Geometry: final body of the model. Coordinates: model frame, mm. A direction names the side the tool comes from. Coordinates: 2 decimals unless noted, no trailing zeros. Order: outer loops, then holes, each group sorted by start corner. A loop starts at its lowest first (then second) coordinate and runs counter-clockwise, first axis right, second up. Notation, with made-up numbers: (-2.5, 44) - (5.5, 44) arc R13 cw to (5.5, 53) - close; hole circle Ø2 at (-2, 47). An arc over 180 degrees is marked (long way). Use a Markdown table: item, result. Add a question column.
```python
from build123d import *

# Parameters (mm, degrees)
SKETCH1_W           = 182
SKETCH1_H           = 137.36
BOSS_EXTRUDE1_DEPTH = 3
SKETCH2_R           = 1.5
CUT_EXTRUDE1_DEPTH  = 4
SKETCH3_R           = 1
CUT_EXTRUDE2_DEPTH  = 4
SKETCH4_W           = 23
SKETCH4_H           = 12.5
CUT_EXTRUDE3_DEPTH  = 4
SKETCH5_R           = 1.35
CUT_EXTRUDE4_DEPTH  = 4
SKETCH6_R           = 1.5
CUT_EXTRUDE5_DEPTH  = 4
CUT_EXTRUDE6_DEPTH  = 4
FILLET1_R           = 7
SKETCH10_R          = 1.5
CUT_EXTRUDE9_DEPTH  = 4
SKETCH11_R          = 1.5
CUT_EXTRUDE10_DEPTH = 4
CUT_EXTRUDE11_REACH = 5
SKETCH13_W          = 12.5
SKETCH13_H          = 23
SKETCH14_R          = 1
CUT_EXTRUDE12_DEPTH = 4
SKETCH15_R          = 2
CUT_EXTRUDE13_DEPTH = 4
SKETCH16_R          = 1.5
CUT_EXTRUDE14_DEPTH = 4


with BuildPart() as part:
    # Sketch1 → Boss-Extrude1 (new body)
    with BuildSketch(Plane(origin=(0, 0, 0), x_dir=(1, 0, 0), z_dir=(0, 1, 0))):
        with Locations((8.068181818, 1013.883570356)):
            Rectangle(SKETCH1_W, SKETCH1_H)
    extrude(amount=BOSS_EXTRUDE1_DEPTH)

    # Sketch2 → Cut-Extrude1 (cut, through all)
    with BuildSketch(Plane.XZ):
        with Locations((95.068181818, -1029.883570356)):
            Circle(SKETCH2_R)
        with Locations((95.068181818, -997.883570356)):
            Circle(SKETCH2_R)
    extrude(amount=-CUT_EXTRUDE1_DEPTH, mode=Mode.SUBTRACT)

    # Sketch3 → Cut-Extrude2 (cut, through all)
    with BuildSketch(Plane(origin=(0, 3, 0), x_dir=(1, 0, 0), z_dir=(0, 1, 0))):
        with Locations((27.328181818, 1076.423570356)):
            Circle(SKETCH3_R)
        with Locations((-0.871818182, 1076.423570356)):
            Circle(SKETCH3_R)
        with Locations((-0.871818182, 951.363570356)):
            Circle(SKETCH3_R)
        with Locations((27.328181818, 951.363570356)):
            Circle(SKETCH3_R)
    extrude(amount=-CUT_EXTRUDE2_DEPTH, mode=Mode.SUBTRACT)

    # Sketch4 → Cut-Extrude3 (cut, through all)
    with BuildSketch(Plane(origin=(0, 3, 0), x_dir=(1, 0, 0), z_dir=(0, 1, 0))):
        with Locations((13.268181818, 951.453570356)):
            Rectangle(SKETCH4_W, SKETCH4_H)
        with Locations((13.268181818, 1076.313570356)):
            Rectangle(SKETCH4_W, SKETCH4_H)
    extrude(amount=-CUT_EXTRUDE3_DEPTH, mode=Mode.SUBTRACT)

    # Sketch5 → Cut-Extrude4 (cut, through all)
    with BuildSketch(Plane.XZ):
        with Locations((77.568181818, -1038.383570356)):
            Circle(SKETCH5_R)
        with Locations((77.668181818, -989.343570356)):
            Circle(SKETCH5_R)
        with Locations((19.568181818, -1038.383570356)):
            Circle(SKETCH5_R)
        with Locations((19.568181818, -989.383570356)):
            Circle(SKETCH5_R)
    extrude(amount=-CUT_EXTRUDE4_DEPTH, mode=Mode.SUBTRACT)

    # Sketch6 → Cut-Extrude5 (cut, through all)
    with BuildSketch(Plane(origin=(0, 3, 0), x_dir=(1, 0, 0), z_dir=(0, 1, 0))):
        with Locations((18.062803793, 1049.383570356)):
            Circle(SKETCH6_R)
        with Locations((-31.937196207, 1049.383570356)):
            Circle(SKETCH6_R)
        with Locations((-31.937196207, 978.387370356)):
            Circle(SKETCH6_R)
        with Locations((18.062803793, 978.387370356)):
            Circle(SKETCH6_R)
    extrude(amount=-CUT_EXTRUDE5_DEPTH, mode=Mode.SUBTRACT)

    # Sketch7 → Cut-Extrude6 (cut, through all)
    with BuildSketch(Plane(origin=(0, 3, 0), x_dir=(1, 0, 0), z_dir=(0, 1, 0))):
        with BuildLine():
            Line((49.068181818, 1063.883570356), (60.068181818, 1063.883570356))
            ThreePointArc((60.068181818, 1063.883570356), (61.482395381, 1063.297783918), (62.068181818, 1061.883570356))
            Line((62.068181818, 1061.883570356), (62.068181818, 965.883570356))
            ThreePointArc((62.068181818, 965.883570356), (61.482395381, 964.469356794), (60.068181818, 963.883570356))
            Line((60.068181818, 963.883570356), (49.068181818, 963.883570356))
            ThreePointArc((49.068181818, 963.883570356), (47.653968256, 964.469356794), (47.068181818, 965.883570356))
            Line((47.068181818, 965.883570356), (47.068181818, 1061.883570356))
            ThreePointArc((47.068181818, 1061.883570356), (47.653968256, 1063.297783918), (49.068181818, 1063.883570356))
        make_face()
        with BuildLine():
            Line((-17.931818182, 1056.563570356), (-57.931818182, 1056.563570356))
            ThreePointArc((-57.931818182, 1056.563570356), (-65.931818182, 1064.563570356), (-57.931818182, 1072.563570356))
            Line((-57.931818182, 1072.563570356), (-17.931818182, 1072.563570356))
            ThreePointArc((-17.931818182, 1072.563570356), (-9.931818182, 1064.563570356), (-17.931818182, 1056.563570356))
        make_face()
        with BuildLine():
            Line((-17.931818182, 955.203570356), (-57.931818182, 955.203570356))
            ThreePointArc((-57.931818182, 955.203570356), (-65.931818182, 963.203570356), (-57.931818182, 971.203570356))
            Line((-57.931818182, 971.203570356), (-17.931818182, 971.203570356))
            ThreePointArc((-17.931818182, 971.203570356), (-9.931818182, 963.203570356), (-17.931818182, 955.203570356))
        make_face()
    extrude(amount=-CUT_EXTRUDE6_DEPTH, mode=Mode.SUBTRACT)

    # Fillet1
    fillet1_edges = [part.edges().sort_by_distance(p)[0] for p in [
        (-82.931818182, 1.5, -1082.563570356),
        (99.068181818, 1.5, -1082.563570356),
        (99.068181818, 1.5, -945.203570356),
        (-82.931818182, 1.5, -945.203570356),
    ]]
    fillet(fillet1_edges, radius=FILLET1_R)

    # Sketch10 → Cut-Extrude9 (cut, through all)
    with BuildSketch(Plane(origin=(0, 3, 0), x_dir=(1, 0, 0), z_dir=(0, 1, 0))):
        with Locations((96.068181818, 1074.563570356)):
            Circle(SKETCH10_R)
        with Locations((81.068181818, 1074.563570356)):
            Circle(SKETCH10_R)
        with Locations((81.068181818, 953.203570356)):
            Circle(SKETCH10_R)
        with Locations((96.068181818, 953.203570356)):
            Circle(SKETCH10_R)
    extrude(amount=-CUT_EXTRUDE9_DEPTH, mode=Mode.SUBTRACT)

    # Sketch11 → Cut-Extrude10 (cut, through all)
    with BuildSketch(Plane.XZ):
        with Locations((-67.845029609, -1046.883570356)):
            Circle(SKETCH11_R)
        with Locations((-67.931818182, -980.883570356)):
            Circle(SKETCH11_R)
    extrude(amount=-CUT_EXTRUDE10_DEPTH, mode=Mode.SUBTRACT)

    # Sketch13 → Cut-Extrude11 (cut, up to next)
    with BuildSketch(Plane.XZ, mode=Mode.PRIVATE) as cut_extrude11_sk1:
        with Locations((-76.681818182, -1008.803570356)):
            Rectangle(SKETCH13_W, SKETCH13_H)
    cut_extrude11_tool1 = extrude(cut_extrude11_sk1.sketch, amount=-CUT_EXTRUDE11_REACH, mode=Mode.PRIVATE) & part.part
    add(cut_extrude11_tool1.solids().sort_by_distance((-76.681818, 0, -1008.80357))[0], mode=Mode.SUBTRACT)

    # Sketch14 → Cut-Extrude12 (cut, through all)
    with BuildSketch(Plane(origin=(0, 3, 0), x_dir=(1, 0, 0), z_dir=(0, 1, 0))):
        with Locations((-76.787040817, 994.553570356)):
            Circle(SKETCH14_R)
        with Locations((-76.787040817, 1022.753570356)):
            Circle(SKETCH14_R)
    extrude(amount=-CUT_EXTRUDE12_DEPTH, mode=Mode.SUBTRACT)

    # Sketch15 → Cut-Extrude13 (cut, through all)
    with BuildSketch(Plane.XZ):
        with Locations((95.068181818, -1042.883570356)):
            Circle(SKETCH15_R)
        with Locations((95.068181818, -984.883570356)):
            Circle(SKETCH15_R)
    extrude(amount=-CUT_EXTRUDE13_DEPTH, mode=Mode.SUBTRACT)

    # Sketch16 → Cut-Extrude14 (cut, through all)
    with BuildSketch(Plane(origin=(0, 3, 0), x_dir=(1, 0, 0), z_dir=(0, 1, 0))):
        with Locations((72.068181818, 1027.563570356)):
            Circle(SKETCH16_R)
        with Locations((72.068181818, 1012.563570356)):
            Circle(SKETCH16_R)
        with Locations((72.068181818, 997.563570356)):
            Circle(SKETCH16_R)
        with Locations((84.068181818, 1007.563570356)):
            Circle(SKETCH16_R)
        with Locations((84.068181818, 1022.563570356)):
            Circle(SKETCH16_R)
        with Locations((84.068181818, 1037.563570356)):
            Circle(SKETCH16_R)
        with Locations((75.068181818, 1062.563570356)):
            Circle(SKETCH16_R)
        with Locations((91.068181818, 1062.563570356)):
            Circle(SKETCH16_R)
        with Locations((83.068181818, 1057.563570356)):
            Circle(SKETCH16_R)
        with Locations((83.068181818, 1067.563570356)):
            Circle(SKETCH16_R)
        with Locations((91.068181818, 965.203570356)):
            Circle(SKETCH16_R)
        with Locations((75.068181818, 965.203570356)):
            Circle(SKETCH16_R)
        with Locations((83.068181818, 970.203570356)):
            Circle(SKETCH16_R)
        with Locations((83.068181818, 960.203570356)):
            Circle(SKETCH16_R)
        with Locations((84.068181818, 992.563570356)):
            Circle(SKETCH16_R)
    extrude(amount=-CUT_EXTRUDE14_DEPTH, mode=Mode.SUBTRACT)


solid = part.part
```
1) First-contact query: pin 1 (1.8 mm diameter, centred on x = 72.07, z = -1012.56, fed in from -Y). Flat tip, straight axial feed; report the tip coordinate or a pass-through.
2) Draft query along X for faces 1 (the cylindrical face through (96.963, 1.521, -947.2)), 2 (the cylindrical face through (-9.934, 1.521, -1064.739)), 3 (the flat face through (7, 3, -1015)). Return one class per face: released by +X, released by -X, zero draft, split by the parting line, or undercut.
3) Section query B-B (x = -64). Return the cut outline in (y, z).
4) Access query for faces 4 (the cylindrical face through (-65.93, 1.52, -1064.39)), 5 (the cylindrical face through (-80.936, 1.521, -1080.459)). Directions: +Z, -Z, +X, -X, +Y, -Y. A direction counts if a zero-diameter tool reaches every point of the face in a straight line with its end or side. Return the directions, or none.
5) Section query C-C (y = 0.95). Give the number of separate pieces and of enclosed holes in the cut face, and give its area (3 significant figures).
6) Section query A-A (x = 52). Return the cut outline in (y, z), and give its area (3 significant figures).
7) Line query: line 1 (Z direction, x = 50, y = 0.3); line 2 (Z direction, x = -20, y = 0.8); line 3 (X direction, y = 2.4, z = -1035). Output: solid intervals per line, ascending. Write a range as from..to.
From the geometry:
| question | item | result |
|---|---|---|
| 1 | pin 1 | passes through |
| 2 | face 1 | released by +X |
| 2 | face 2 | undercut |
| 2 | face 3 | zero draft |
| 3 | outline | (0, -1082.56) - (3, -1082.56) - (3, -1069.78) - (0, -1069.78) - close; (0, -1059.35) - (3, -1059.35) - (3, -968.42) - (0, -968.42) - close; (0, -957.99) - (3, -957.99) - (3, -945.2) - (0, -945.2) - close |
| 4 | face 4 | +Y, -Y |
| 4 | face 5 | -Z, -X, +Y, -Y |
| 5 | separate pieces | 1 |
| 5 | enclosed holes | 42 |
| 5 | area | 20,700 mm^2 |
| 6 | outline | (0, -1082.56) - (3, -1082.56) - (3, -1063.88) - (0, -1063.88) - close; (0, -963.88) - (3, -963.88) - (3, -945.2) - (0, -945.2) - close |
| 6 | area | 112 mm^2 |
| 7 | line 1 | z = -1082.56..-1063.88, -963.88..-945.2 |
| 7 | line 2 | z = -1082.56..-1072.56, -1056.56..-971.2, -955.2..-945.2 |
| 7 | line 3 | x = -82.93..47.07, 62.07..99.07 |
